The listing builds one solid part. Answer for the finished solid, in the listing's coordinates (mm). Coordinates: 2 decimals unless noted, no trailing zeros. Loops run counter-clockwise (first coordinate to the right, second up) from the corner with the lowest first, then second, coordinate; pieces in that order, holes last. Notation, with made-up numbers: M 29,41.25 L 68,41.25 A11 cw 68,48.25 Z; hole C 59,81 d11. An arc over 180 degrees is marked long. Return JSON: item names as keys, results as strings. Group by question number.
1. Section B-B (x = -2) is taken. Write down the section's boundary in (y, z), then the cut area to 3 significant figures.
2. Section C-C (y = -7) is taken. Write down the section's boundary in (x, z), then the cut area to 3 significant figures.
3. Straight lines are drawn through the part: L1, parallel to Y at x = 10, z = 1.8; L2, parallel to Y at x = -10, z = 1.25; L3, parallel to Y at x = 9, z = 2.25. For each, find the intervals that lie inside material, in ascending order. Write a range as from..to.
4. Section D-D (x = 10) is taken. Write down the section's boundary in (y, z).
5. Section A-A (y = 7) is taken. Write down the section's boundary in (x, z), then the cut area to 3 significant figures.
6. Given P1, Ø8, axis at x = -15, y = -9, coming from the -Z side, flat-ended and moving along its own axis, determine where the tip first touches the part or whether it passes through.
```python
from build123d import *

# Parameters (mm, degrees)
SKETCH_1_R      = 1.6
EXTRUDE_1_DEPTH = 2.5
FILLET_2_R      = 2


with BuildPart() as part:
    # 草图1 → 凸台-拉伸1 (new body)
    with BuildSketch(Plane.XY):
        Polygon((-19, 17), (19, 17), (19, -26), (-13, -26), (-13, -17), (-19, -17), align=None)
        with Locations((10, 7)):
            Circle(SKETCH_1_R, mode=Mode.SUBTRACT)
        with Locations((-10, 7)):
            Circle(SKETCH_1_R, mode=Mode.SUBTRACT)
        with Locations((10, -22.5)):
            Circle(SKETCH_1_R, mode=Mode.SUBTRACT)
        with Locations((10, -7)):
            Circle(SKETCH_1_R, mode=Mode.SUBTRACT)
        with Locations((-2, -19)):
            Circle(SKETCH_1_R, mode=Mode.SUBTRACT)
    extrude(amount=EXTRUDE_1_DEPTH)

    # 圆角2
    fillet_2_edges = [part.edges().sort_by_distance(p)[0] for p in [
        (-19, 17, 1.25),
        (19, 17, 1.25),
        (19, -26, 1.25),
        (-13, -26, 1.25),
        (-13, -17, 1.25),
        (-19, -17, 1.25),
    ]]
    fillet(fillet_2_edges, radius=FILLET_2_R)


solid = part.part
```
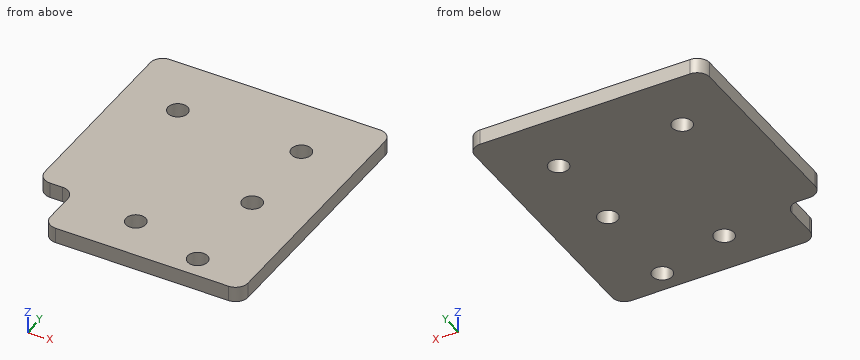
Worked out:
{
 "1": {"outline": "M -26,0 L -20.6,0 L -20.6,2.5 L -26,2.5 Z; M -17.4,0 L 17,0 L 17,2.5 L -17.4,2.5 Z", "area": "99.5 mm^2"},
 "2": {"outline": "M -19,0 L 8.4,0 L 8.4,2.5 L -19,2.5 Z; M 11.6,0 L 19,0 L 19,2.5 L 11.6,2.5 Z", "area": "87.0 mm^2"},
 "3": {"L1": "-26..-24.1, -20.9..-8.6, -5.4..5.4, 8.6..17", "L2": "-26..5.4, 8.6..17", "L3": "-26..-23.75, -21.25..-8.25, -5.75..5.75, 8.25..17"},
 "4": {"outline": "M -26,0 L -24.1,0 L -24.1,2.5 L -26,2.5 Z; M -20.9,0 L -8.6,0 L -8.6,2.5 L -20.9,2.5 Z; M -5.4,0 L 5.4,0 L 5.4,2.5 L -5.4,2.5 Z; M 8.6,0 L 17,0 L 17,2.5 L 8.6,2.5 Z"},
 "5": {"outline": "M -19,0 L -11.6,0 L -11.6,2.5 L -19,2.5 Z; M -8.4,0 L 8.4,0 L 8.4,2.5 L -8.4,2.5 Z; M 11.6,0 L 19,0 L 19,2.5 L 11.6,2.5 Z", "area": "79.0 mm^2"},
 "6": {"P1": "z = 0"}
}
